Autodesk Fusion 360 part; units mm, degrees
sketch "Sketch1" plane through (0, 0, 0) normal (0, 0, 1) x (1, 0, 0)
  line L0 (0, 0) -> (100, 0) construction
  line L1 (100, 0) -> (0, 0) construction
  circle A0 centre (0, 0) radius 20
  circle A1 centre (100, 0) radius 30
  line L2 (-2, 19.8997) -> (97, 29.8496)
  line L3 (-2, -19.8997) -> (97, -29.8496)
  circle A2 centre (0, 0) radius 10
  circle A3 centre (100, 0) radius 10
  dimension "d1" = 100
  dimension "d2" = 40
  dimension "d3" = 60
  dimension "d4" = 20
  dimension "d5" = 20
extrude "Extrude1" add sketch "Sketch1" along normal blind 20 contours A0 | A1 | A2 | A3 makes body 1 at (19.9751, 0.9969, 6.6667) makes body 2 at (129.8509, -2.987, 6.6667)
extrude "Extrude2" add sketch "Sketch1" along normal blind 10 contours A0 A1 L2 L3 bodies 1 2
hole "Hole1" at (100, 0, 0) direction (0, 0, 1) diameter 20 depth 40 tip angle 180 bodies 1
hole "Hole2" at (0, 0, 0) direction (0, 0, 1) diameter 20 end through all bodies 1 1
Geometry: final body of the model. Coordinates: model frame, mm. A direction names the side the tool comes from. Round coordinates to 2 decimals unless told otherwise and drop trailing zeros. Order: outer loops, then holes, each group sorted by start corner. A loop starts at its lowest first (then second) coordinate and runs counter-clockwise, first axis right, second up.
Q1. Section B-B, the plane y = -3. Output: boundary loops of the cut face in (x, z).
Result sheet:
outline: (-19.77, 0) - (-9.54, 0) - (-9.54, 20) - (-19.77, 20) - close; (9.54, 0) - (90.46, 0) - (90.46, 20) - (70.15, 20) - (70.15, 10) - (19.77, 10) - (19.77, 20) - (9.54, 20) - close; (109.54, 0) - (129.85, 0) - (129.85, 20) - (109.54, 20) - close
Q2. Section C-C, the plane z = 5.25. Output: boundary loops of the cut face in (x, y), and give its area (3 significant figures).
Result sheet:
outline: (-2, -19.9) - (97, -29.85) arc R30 ccw (long way) to (97, 29.85) - (-2, 19.9) arc R20 ccw to start; hole circle Ø20 at (0, 0); hole circle Ø20 at (100, 0)
area: 6,440 mm2
Q3. Mould query, pull axis Y, two halves, no side actions, for faces 1 (the face through (-5, 9, 20)), 2 (the face through (9.76, -2.17, 10.14)), 3 (the face through (-19.98, -0.88, 12.08)). Classes: released by +Y, released by -Y, zero draft, split by the parting line, or undercut.
Result sheet:
face 1: zero draft
face 2: undercut
face 3: split by the parting line
Q4. Section D-D, the plane x = 0. Output: boundary loops of the cut face in (y, z).
Result sheet:
outline: (-20.1, 0) - (-10, 0) - (-10, 20) - (-20, 20) - (-20, 10) - (-20.1, 10) - close; (10, 0) - (20.1, 0) - (20.1, 10) - (20, 10) - (20, 20) - (10, 20) - close
Q5. Material intervals for probe 1 along X at (y, z) = (0, 15); probe 2 along X at (y, z) = (0, 8.5); probe 3 along X at (y, z) = (8, 16.5), sorted ascending.
Result sheet:
probe 1: x = -20 to -10, 10 to 20, 70 to 90, 110 to 130
probe 2: x = -20 to -10, 10 to 90, 110 to 130
probe 3: x = -18.33 to -6, 6 to 18.33, 71.09 to 94, 106 to 128.91
Q6. Pin query (flat end, axial travel): pin 1 (6 mm diameter, centred on x = 32.5, y = 12, fed in from +Z); pin 2 (6 mm diameter, centred on x = 34, z = 6.5, fed in from -Y); pin 3 (16 mm diameter, centred on x = 100, y = 0, fed in from +Z); pin 4 (8 mm diameter, centred on x = 58.5, z = 8.5, fed in from -Y). Return the tip coordinate at first contact, or that it passes through.
Result sheet:
pin 1: stops at z = 10
pin 2: stops at y = -23.82
pin 3: passes through
pin 4: stops at y = -26.38
Q7. Section A-A, the plane x = 100. Output: boundary loops of the cut face in (y, z), and give its area (3 significant figures).
Result sheet:
outline: (-30, 0) - (-10, 0) - (-10, 20) - (-30, 20) - close; (10, 0) - (30, 0) - (30, 20) - (10, 20) - close
area: 800 mm2
Q8. Access query for faces 4 (the face through (90.085, -1.302, 10.14)), 5 (the face through (128.615, -9.011, 12.082)). Directions: +Z, -Z, +X, -X, +Y, -Y. A direction counts if a zero-diameter tool reaches every point of the face in a straight line with its end or side. Return the directions, or none.
Result sheet:
face 4: +Z, -Z
face 5: +Z
